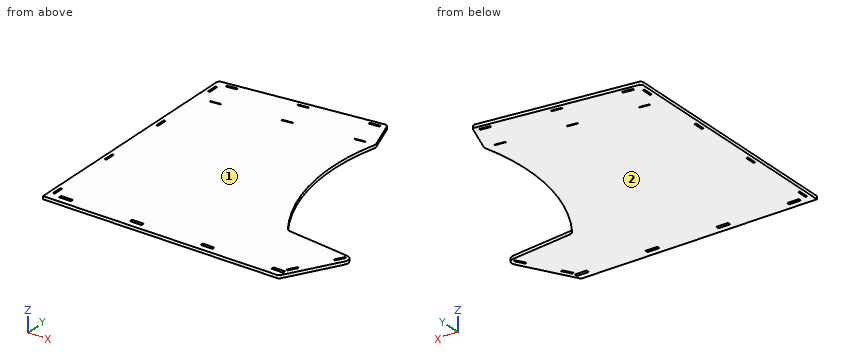
Autodesk Inventor part; units mm, degrees
ref_plane "YZ Plane" through (0, 0, 0) normal (1, 0, 0) x (0, 1, 0)
ref_plane "XZ Plane" through (0, 0, 0) normal (0, 1, 0) x (-1, 0, 0)
ref_plane "XY Plane" through (0, 0, 0) normal (0, 0, 1) x (1, 0, 0)
sketch "Sketch1" plane through (0, 0, 0) normal (0, 0, 1) x (1, 0, 0)
  line L0 (0, 0) -> (794.2265, 0)
  line L1 (0, 0) -> (0, 821.1016)
  line L2 (8.8381, 831.0339) -> (522.0969, 891.0755)
  line L3 (802.8868, 5) -> (900.3166, 173.7534)
  line L4 (532.6762, 884.5066) -> (567.9402, 785.7674)
  arc A0 (532.6762, 884.5066) -> (522.0969, 891.0755) centre (523.2588, 881.1432) ccw
  arc A1 (8.8381, 831.0339) -> (0, 821.1016) centre (10, 821.1016) ccw
  arc A2 (794.2265, 0) -> (802.8868, 5) centre (794.2265, 10) ccw
  line L5 (265.4675, 861.0547) -> (267.2222, 846.0547) construction
  line L6 (14.3861, 816.4776) -> (535.2127, 877.4045) construction
  line L7 (20, 820.1548) -> (531.512, 879.9921) construction
  line L8 (531.512, 879.9921) -> (532.2091, 874.0327) construction
  line L9 (532.2091, 874.0327) -> (20.6971, 814.1954) construction
  line L10 (20.6971, 814.1954) -> (20, 820.1548) construction
  line L11 (34.8984, 821.8976) -> (35.5955, 815.9383)
  line L12 (69.6614, 825.9643) -> (70.3585, 820.0049)
  line L13 (481.8506, 874.1826) -> (482.5478, 868.2233)
  line L14 (516.6136, 878.2492) -> (517.3107, 872.2899)
  line L15 (34.8984, 821.8976) -> (69.6614, 825.9643)
  line L16 (70.3585, 820.0049) -> (35.5955, 815.9383)
  line L17 (516.6136, 878.2492) -> (481.8506, 874.1826)
  line L18 (482.5478, 868.2233) -> (517.3107, 872.2899)
  line L19 (20.3486, 817.1751) -> (531.8605, 877.0124) construction
  line L20 (275.756, 850.0734) -> (276.1046, 847.0938) construction
  line L21 (569.7285, 780.7603) -> (0, 714.1128) construction
  line L22 (49.9711, 721.4687) -> (50.3197, 718.489)
  line L23 (84.734, 725.5353) -> (85.0826, 722.5557)
  line L24 (501.8894, 774.3347) -> (502.238, 771.355)
  line L25 (536.6524, 778.4013) -> (537.001, 775.4216)
  line L26 (49.9711, 721.4687) -> (84.734, 725.5353)
  line L27 (85.0826, 722.5557) -> (50.3197, 718.489)
  line L28 (536.6524, 778.4013) -> (501.8894, 774.3347)
  line L29 (502.238, 771.355) -> (537.001, 775.4216)
  line L30 (20, 719.4729) -> (566.2749, 783.3768) construction
  line L31 (566.2749, 783.3768) -> (566.9721, 777.4174) construction
  line L32 (566.9721, 777.4174) -> (20.6971, 713.5135) construction
  line L33 (20.6971, 713.5135) -> (20, 719.4729) construction
  line L34 (15, 0) -> (15, 541.5516) construction
  line L35 (12, 800) -> (18, 800)
  line L36 (18, 800) -> (18, 765)
  line L37 (18, 765) -> (12, 765)
  line L38 (12, 765) -> (12, 800)
  line L39 (12, 555) -> (18, 555)
  line L40 (18, 555) -> (18, 520)
  line L41 (18, 520) -> (12, 520)
  line L42 (12, 520) -> (12, 555)
  line L43 (12, 310) -> (18, 310)
  line L44 (18, 310) -> (18, 275)
  line L45 (18, 275) -> (12, 275)
  line L46 (12, 275) -> (12, 310)
  line L47 (12, 65) -> (18, 65)
  line L48 (18, 65) -> (18, 30)
  line L49 (18, 30) -> (12, 30)
  line L50 (12, 30) -> (12, 65)
  line L51 (31.6599, 656.3688) -> (531.6599, 656.3688) construction
  line L52 (531.6599, 656.3688) -> (531.6599, 36.3688) construction
  line L53 (531.6599, 36.3688) -> (31.6599, 36.3688) construction
  line L54 (31.6599, 36.3688) -> (31.6599, 656.3688) construction
  line L55 (885.379, 203.6109) -> (674.5616, 228.909)
  arc A3 (568.4993, 774.1544) -> (660.278, 237.7109) centre (1221.1056, 609.7342) ccw
  line L56 (40, 30) -> (80, 30)
  line L57 (80, 30) -> (80, 20)
  line L58 (80, 20) -> (40, 20)
  line L59 (40, 20) -> (40, 30)
  line L60 (280, 30) -> (320, 30)
  line L61 (320, 30) -> (320, 20)
  line L62 (320, 20) -> (280, 20)
  line L63 (280, 20) -> (280, 30)
  line L64 (520, 30) -> (560, 30)
  line L65 (560, 30) -> (560, 20)
  line L66 (560, 20) -> (520, 20)
  line L67 (520, 20) -> (520, 30)
  line L68 (760, 30) -> (800, 30)
  line L69 (800, 30) -> (800, 20)
  line L70 (800, 20) -> (760, 20)
  line L71 (760, 20) -> (760, 30)
  arc A4 (900.3166, 173.7534) -> (885.379, 203.6109) centre (882.9961, 183.7534) ccw
  arc A5 (660.278, 237.7109) -> (674.5616, 228.909) centre (676.9445, 248.7665) ccw
  arc A6 (568.4993, 774.1544) -> (567.9402, 785.7674) centre (549.1054, 779.0406) ccw
  line L72 (52.2799, 823.9309) -> (52.6284, 820.9513) construction
  line L73 (258.6126, 846.0051) -> (259.0716, 842.0808)
  line L74 (293.3755, 850.0717) -> (293.8346, 846.1474)
  line L75 (258.6126, 846.0051) -> (293.3755, 850.0717)
  line L76 (293.8346, 846.1474) -> (259.0716, 842.0808)
  line L77 (275.994, 848.0384) -> (276.3426, 845.0587) construction
  line L78 (519.2709, 776.368) -> (519.4452, 774.8781)
  line L79 (310.1966, 751.9102) -> (310.5452, 748.9305)
  line L80 (275.4337, 747.8436) -> (275.7822, 744.8639)
  line L81 (310.1966, 751.9102) -> (275.4337, 747.8436)
  line L82 (275.7822, 744.8639) -> (310.5452, 748.9305)
  line L83 (292.8151, 749.8769) -> (292.9894, 748.3871)
  line L84 (796.8079, 40.4711) -> (802.0041, 37.4711)
  line L85 (802.0041, 37.4711) -> (819.5041, 67.782)
  line L86 (819.5041, 67.782) -> (814.3079, 70.782)
  line L87 (814.3079, 70.782) -> (796.8079, 40.4711)
  line L88 (873.5041, 161.3128) -> (868.3079, 164.3128)
  line L89 (868.3079, 164.3128) -> (885.8079, 194.6237)
  line L90 (885.8079, 194.6237) -> (891.0041, 191.6237)
  line L91 (891.0041, 191.6237) -> (873.5041, 161.3128)
  line L92 (840.6385, 70.388) -> (823.318, 80.388) construction
  line L93 (892.9961, 201.0739) -> (776.906, 0) construction
  line L94 (799.406, 38.9711) -> (888.406, 193.1237) construction
  line L95 (843.906, 116.0474) -> (847.4398, 114.0072) construction
  line L96 (797.981, 30.503) -> (792.7848, 33.503) construction
  line L97 (796.8079, 40.4711) -> (792.7848, 33.503) construction
  line L98 (801.8634, 37.2275) -> (797.981, 30.503) construction
  line L99 (819.5041, 67.782) -> (873.5041, 161.3128) construction
  line L100 (868.3079, 164.3128) -> (814.3079, 70.782) construction
  line L101 (885.8079, 194.6237) -> (890.2848, 202.3779) construction
  line L102 (891.0041, 191.6237) -> (895.481, 199.3779) construction
  line L103 (890.2848, 202.3779) -> (895.481, 199.3779) construction
  line L104 (569.0823, 778.0788) -> (665.4701, 230) construction
  line L105 (665.4701, 230) -> (546.1008, 230) construction
  line L106 (569.0823, 778.0788) -> (515.1258, 778.0788) construction
  line L107 (509.3451, 770.6761) -> (604.6809, 230) construction
  point P0 (800, 0)
  point P1 (0, 830)
  point P2 (530, 892)
  point P3 (570, 780)
  point P4 (915.4701, 200)
  point P5 (570, 780)
  point P6 (15, 65)
  point P7 (84.9083, 724.0455)
  point P8 (502.0637, 772.8448)
  point P9 (20.3486, 716.4932)
  point P10 (275.6079, 746.3538)
  dimension "d0" = 830
  dimension "d1" = 62
  dimension "d2" = 50
  dimension "d3" = 800
  dimension "d9" = 530
  dimension "d10" = 570
  dimension "d13" = 10
  dimension "d16" = 15
  dimension "d17" = 6
  dimension "d18" = 515
  dimension "d19" = 35
  dimension "d20" = 15
  dimension "d21" = 15
  dimension "d22" = 35
  dimension "d23" = 415
  dimension "d24" = 35
  dimension "d25" = 35
  dimension "d27" = 6
  dimension "d28" = 550
  dimension "d31" = 15
  dimension "d32" = 35
  dimension "d33" = 6
  dimension "d34" = 30
  dimension "d35" = 210
  dimension "d36" = 210
  dimension "d37" = 210
  dimension "d38" = 30
  dimension "d39" = 30
  dimension "d40" = 420
  dimension "d42" = 20
  dimension "d48" = 3
  dimension "d50" = 5
  dimension "d51" = 100
  dimension "d58" = 500
  dimension "d59" = 620
  dimension "d60" = 200
  dimension "d61" = 230
  dimension "d62" = 250
  dimension "d63" = 10
  dimension "d64" = 40
  dimension "d65" = 200
  dimension "d66" = 200
  dimension "d67" = 200
  dimension "d68" = 40
  dimension "d69" = 20
  dimension "d72" = 20
  dimension "d73" = 35
  dimension "d74" = 20
  dimension "d75" = 20
  dimension "d76" = 10
  dimension "d77" = 35
  dimension "d78" = 192
  dimension "d79" = 193
  dimension "d80" = 673
  dimension "d84" = 22
  dimension "d85" = 190
  dimension "d86" = 190
  dimension "d87" = 6
  dimension "d88" = 35
  dimension "d89" = 20
  dimension "d90" = 120
  dimension "d91" = 45
  dimension "d92" = 108
  dimension "d93" = 195
extrude "Extrusion6" add sketch "Sketch1" along normal blind 10
properties part number "ladoA" material "Wood (Oak)"
Work out the finished part from the listing and answer in its coordinate system (mm). Face numbers are marked on the shaded views. Give positions to 0.01 mm unless a question says otherwise; leave off trailing zeros. Order: outer loops, then holes, each group sorted by start corner. A loop starts at its lowest first (then second) coordinate and runs counter-clockwise, first axis right, second up. Notation, with made-up numbers: M -31.5,53 L 16.5,53 A37 cw 16.5,89 Z; hole C 70,13.5 d9. An arc over 180 degrees is marked long. Return JSON: item names as keys, results as strings.
1) Section C-C, the plane x = 175.5 is taken. Write down the section's boundary in (y, z), plus the area to 3 significant figures.
Resolved:
{"outline": "M 0,0 L 850.53,0 L 850.53,10 L 0,10 Z", "area": "8,510 mm^2"}
2) Straight lines are drawn through the part: line 1 along Y through (x, z) = (363.5, 0.5); line 2 along X through (y, z) = (186.5, 5.75); line 3 along X through (y, z) = (794, 3.5). For each, find the intervals that lie inside material, in ascending order. Write a range as [from, to].
Resolved:
{"line 1": "[0, 872.52]", "line 2": "[0, 881.12], [888.05, 902.81]", "line 3": "[0, 12], [18, 565]"}
3) Each of these flat-tipped pins is pushed along its axis until it touches: pin 1 (5 mm diameter, centred on y = 285, z = 6.5, fed in from +X); pin 2 (5 mm diameter, centred on x = 528.5, z = 1, fed in from +Y); pin 3 (1.8 mm diameter, centred on x = 13.5, z = 5.5, fed in from +Y). Where does it stop, or does it pass through?
Resolved:
{"pin 1": "x = 633.02", "pin 2": "y = 890.76", "pin 3": "y = 831.68"}
4) Section B-B, the plane y = 638.5 is taken. Write down the section's boundary in (x, z), plus the area to 3 significant figures.
Resolved:
{"outline": "M 0,0 L 548.72,0 L 548.72,10 L 0,10 Z", "area": "5,490 mm^2"}
5) For a pull along Z with two mould halves and no side action, classify the marked faces 1 and 2 as +Z half, -Z half, draft (parallel to the pull), parting line (faces both ways), or undercut.
Resolved:
{"face 1": "+Z half", "face 2": "-Z half"}
6) Section A-A, the plane z = 6.75 is taken. Give the number of separate pieces and of enclosed holes in the cut face, plus the area to 3 significant figures.
Resolved:
{"separate pieces": "1", "enclosed holes": "16", "area": "553,000 mm^2"}
